Build history of the part. All positions in model axes, mm. Face numbers are marked on the shaded views. A direction names the side the tool comes from. Coordinates: 2 decimals unless noted, no trailing zeros. Write each loop counter-clockwise with the first axis right and the second up, starting at its lowest first coordinate (ties: lowest second). Pieces come first, ordered by that corner, then holes.
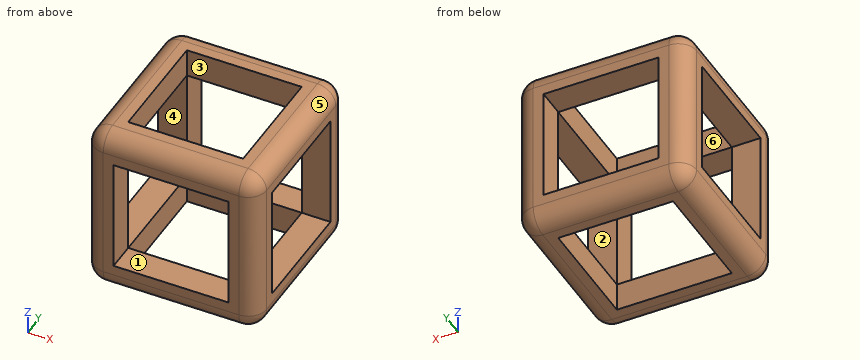
```python
from build123d import *

# Parameters (mm, degrees)
F0_W      = 19.05
F0_H      = 19.05
F1_DEPTH  = 19.05
F2_R      = 2.032
F3_W      = 12.7
F3_H      = 12.7
F4_DEPTH  = 3.302
F5_W      = 6.35
F5_H      = 12.7
F6_DEPTH  = 3.302
F7_W      = 6.35
F7_H      = 12.7
F8_DEPTH  = 3.302
F9_W      = 6.35
F9_H      = 12.7
F10_DEPTH = 3.302
F11_W     = 6.35
F11_H     = 12.7
F12_DEPTH = 3.302
F13_W     = 6.35
F13_H     = 12.7
F14_DEPTH = 41.148


with BuildPart() as f1:
    # F0 (on Top) → F1 (new body)
    with BuildSketch(Plane.XY):
        Rectangle(F0_W, F0_H)
    extrude(amount=F1_DEPTH)

    # F2
    f2_edges = [f1.edges().sort_by_distance(p)[0] for p in [
        (-9.525, 0, 19.05),
        (0, -9.525, 19.05),
        (9.525, 0, 19.05),
        (0, 9.525, 19.05),
        (-9.525, 9.525, 9.525),
        (-9.525, -9.525, 9.525),
        (-9.525, 0, 0),
        (9.525, 9.525, 9.525),
        (0, 9.525, 0),
        (9.525, -9.525, 9.525),
        (0, -9.525, 0),
        (9.525, 0, 0),
    ]]
    fillet(f2_edges, radius=F2_R)

    # F3 (on face) → F4 (cut)
    with BuildSketch(Plane.XY.offset(19.05)):
        Rectangle(F3_W, F3_H)
    extrude(amount=-F4_DEPTH, mode=Mode.SUBTRACT)

    # F5 (on face) → F6 (cut)
    with BuildSketch(Plane(origin=(-9.525, 0, 0), x_dir=(0, -1, 0), z_dir=(-1, 0, 0))):
        with Locations((3.175, 9.525)):
            Rectangle(F5_W, F5_H)
        with Locations((-3.175, 9.525)):
            Rectangle(F5_W, F5_H)
    extrude(amount=-F6_DEPTH, mode=Mode.SUBTRACT)

    # F7 (on face) → F8 (cut)
    with BuildSketch(Plane.YZ.offset(9.525)):
        with Locations((3.175, 9.525)):
            Rectangle(F7_W, F7_H)
        with Locations((-3.175, 9.525)):
            Rectangle(F7_W, F7_H)
    extrude(amount=-F8_DEPTH, mode=Mode.SUBTRACT)

    # F9 (on face) → F10 (cut)
    with BuildSketch(Plane.XZ.offset(9.525)):
        with Locations((3.175, 9.525)):
            Rectangle(F9_W, F9_H)
        with Locations((-3.175, 9.525)):
            Rectangle(F9_W, F9_H)
    extrude(amount=-F10_DEPTH, mode=Mode.SUBTRACT)

    # F11 (on face) → F12 (cut)
    with BuildSketch(Plane(origin=(0, 9.525, 0), x_dir=(-1, 0, 0), z_dir=(0, 1, 0))):
        with Locations((-3.175, 9.525)):
            Rectangle(F11_W, F11_H)
        with Locations((3.175, 9.525)):
            Rectangle(F11_W, F11_H)
    extrude(amount=-F12_DEPTH, mode=Mode.SUBTRACT)

    # F13 (on face) → F14 (cut)
    with BuildSketch(Plane(origin=(0, 0, 0), x_dir=(1, 0, 0), z_dir=(0, 0, -1))):
        with Locations((3.175, 0)):
            Rectangle(F13_W, F13_H)
        with Locations((-3.175, 0)):
            Rectangle(F13_W, F13_H)
    extrude(amount=-F14_DEPTH, mode=Mode.SUBTRACT)


solid = f1.part
```
1. 3-axis set-ups, long thin cutter, end or side, ignore diameter. For the marked faces 1, 2 and 3: which of +Z, -Z, +X, -X, +Y, -Y reach the whole face in a straight line?
Computed values:
face 1: +Y, -Y
face 2: +X, -X
face 3: +Z, -Z
2. Saw through at B-B on z = 15.5. List the corners of the cut face in (x, y) (3 decimals).
Computed values:
outline: (-9.525, -7.493) arc R2.032 ccw to (-7.493, -9.525) - (-6.35, -9.525) - (-6.35, -6.35) - (-9.525, -6.35) - close; (-9.525, 6.35) - (-6.35, 6.35) - (-6.35, 9.525) - (-7.493, 9.525) arc R2.032 ccw to (-9.525, 7.493) - close; (6.35, -9.525) - (7.493, -9.525) arc R2.032 ccw to (9.525, -7.493) - (9.525, -6.35) - (6.35, -6.35) - close; (6.35, 6.35) - (9.525, 6.35) - (9.525, 7.493) arc R2.032 ccw to (7.493, 9.525) - (6.35, 9.525) - close
3. Saw through at D-D on y = 7. List the corners of the cut face in (x, z) (3 decimals).
Computed values:
outline: (-9.525, 2.032) arc R2.032 ccw to (-7.493, 0) - (7.493, 0) arc R2.032 ccw to (9.525, 2.032) - (9.525, 17.018) arc R2.032 ccw to (7.493, 19.05) - (-7.493, 19.05) arc R2.032 ccw to (-9.525, 17.018) - close; hole (-6.35, 3.175) - (6.35, 3.175) - (6.35, 15.875) - (-6.35, 15.875) - close
4. Saw through at A-A on y = -1.25. List the corners of the cut face in (x, z) (3 decimals), plus the area to 3 significant figures.
Computed values:
outline: (-9.525, 2.032) arc R2.032 ccw to (-7.493, 0) - (-6.35, 0) - (-6.35, 3.175) - (-9.525, 3.175) - close; (-9.525, 15.875) - (-6.35, 15.875) - (-6.35, 19.05) - (-7.493, 19.05) arc R2.032 ccw to (-9.525, 17.018) - close; (6.35, 0) - (7.493, 0) arc R2.032 ccw to (9.525, 2.032) - (9.525, 3.175) - (6.35, 3.175) - close; (6.35, 15.875) - (9.525, 15.875) - (9.525, 17.018) arc R2.032 ccw to (7.493, 19.05) - (6.35, 19.05) - close
area: 36.8 mm2
5. Mould opens along X. For the marked faces 4, 5 and 6 say: +X half, -X half, draft (parallel to the pull), parting line (faces both ways), or undercut.
Computed values:
face 4: draft
face 5: +X half
face 6: undercut
6. Flat gauge pins, fed straight in: pin 1 (1.6 mm diameter, centred on y = 2, z = 18, fed in from -X); pin 2 (1 mm diameter, centred on y = 1.5, z = 1, fed in from +X); pin 3 (1.6 mm diameter, centred on x = -8.5, y = -1, fed in from -Z). Where does each tip first touch, or does it go through?
Computed values:
pin 1: stops at x = -9.52
pin 2: stops at x = 9.45
pin 3: stops at z = 0.01
7. Saw through at C-C on x = 8. List the corners of the cut face in (y, z) (3 decimals), plus the area to 3 significant figures.
Computed values:
outline: (-9.461, 2.032) arc R1.968 ccw to (-7.493, 0.064) - (7.493, 0.064) arc R1.968 ccw to (9.461, 2.032) - (9.461, 17.018) arc R1.968 ccw to (7.493, 18.986) - (-7.493, 18.986) arc R1.968 ccw to (-9.461, 17.018) - close; hole (-6.35, 3.175) - (6.35, 3.175) - (6.35, 15.875) - (-6.35, 15.875) - close
area: 193 mm2
8. Probe line 1 along X through (y, z) = (7, 8.5) (3 decimals); line 2 along Z through (x, y) = (6.5, -0.25) (3 decimals). List the from-to ranges inside material, lowest first.
Computed values:
line 1: x = -9.525 to -6.35, 6.35 to 9.525
line 2: z = 0 to 3.175, 15.875 to 19.05
